from build123d import *

# Parameters (mm, degrees)
SKETCH_R        = 1.4
PAD_DEPTH       = 2
SKETCH001_W     = 86
SKETCH001_H     = 4
PAD001_DEPTH    = 55
FILLET_R        = 2
FILLET001_R     = 2
FILLET002_R     = 1
FILLET003_R     = 1
FILLET004_R     = 1
SKETCH002_R     = 1.4
POCKET_DEPTH    = 5
SKETCH003_W     = 15
SKETCH003_H     = 20
PAD002_DEPTH    = 6.85
SKETCH004_R     = 1.4
POCKET001_DEPTH = 15
SKETCH005_R     = 1.4
POCKET002_DEPTH = 20
SKETCH006_W     = 5
SKETCH006_H     = 5
PAD003_DEPTH    = 5
SKETCH007_R     = 1.4
POCKET003_DEPTH = 5
SKETCH008_R     = 1.4
POCKET004_DEPTH = 5
SKETCH009_R     = 1.4
POCKET005_DEPTH = 4


with BuildPart() as part:
    # Sketch → Pad (new body)
    with BuildSketch(Plane.XY):
        with BuildLine():
            ThreePointArc((-41, 25), (-42.414214, 24.414214), (-43, 23))
            Line((-43, -23), (-43, 23))
            ThreePointArc((-43, -23), (-42.414214, -24.414214), (-41, -25))
            Line((41, -25), (-41, -25))
            ThreePointArc((41, -25), (42.414214, -24.414214), (43, -23))
            Line((43, 23), (43, -23))
            ThreePointArc((43, 23), (42.414214, 24.414214), (41, 25))
            Line((-41, 25), (41, 25))
        make_face()
        with Locations((0, 7)):
            Circle(SKETCH_R, mode=Mode.SUBTRACT)
        with Locations((0, -17)):
            Circle(SKETCH_R, mode=Mode.SUBTRACT)
    extrude(amount=PAD_DEPTH)

    # Sketch001 (on Face12 of Pad) → Pad001 (join)
    with BuildSketch(Plane.XY.offset(2)):
        with Locations((0, 1)):
            Rectangle(SKETCH001_W, SKETCH001_H)
    extrude(amount=PAD001_DEPTH)

    # Fillet
    fillet_edges = [part.edges().sort_by_distance(p)[0] for p in [
        (-43, 1, 57),
    ]]
    fillet(fillet_edges, radius=FILLET_R)

    # Fillet001
    fillet001_edges = [part.edges().sort_by_distance(p)[0] for p in [
        (43, 1, 57),
    ]]
    fillet(fillet001_edges, radius=FILLET001_R)

    # Fillet002
    fillet002_edges = [part.edges().sort_by_distance(p)[0] for p in [
        (-43, 3, 28.5),
    ]]
    fillet(fillet002_edges, radius=FILLET002_R)

    # Fillet003
    fillet003_edges = [part.edges().sort_by_distance(p)[0] for p in [
        (-43, -1, 28.5),
    ]]
    fillet(fillet003_edges, radius=FILLET003_R)

    # Fillet004
    fillet004_edges = [part.edges().sort_by_distance(p)[0] for p in [
        (-43, 0, 0),
    ]]
    fillet(fillet004_edges, radius=FILLET004_R)

    # Sketch002 (on Face12 of Fillet004) → Pocket (cut)
    with BuildSketch(Plane(origin=(0, 3, 0), x_dir=(-1, 0, 0), z_dir=(0, 1, 0))):
        with Locations((-27.5, 24)):
            Circle(SKETCH002_R)
        with Locations((27.5, 24)):
            Circle(SKETCH002_R)
    extrude(amount=-POCKET_DEPTH, mode=Mode.SUBTRACT)

    # Sketch003 (on Face6 of Pocket) → Pad002 (join)
    with BuildSketch(Plane.XY.offset(2)):
        with Locations((-23.5, -11)):
            Rectangle(SKETCH003_W, SKETCH003_H)
        with Locations((23.5, -11)):
            Rectangle(SKETCH003_W, SKETCH003_H)
    extrude(amount=PAD002_DEPTH)

    # Sketch004 (on Face23 of Pad002) → Pocket001 (cut)
    with BuildSketch(Plane(origin=(-31, 0, 0), x_dir=(0, -1, 0), z_dir=(-1, 0, 0))):
        with Locations((6, 5)):
            Circle(SKETCH004_R)
        with Locations((16, 5)):
            Circle(SKETCH004_R)
    extrude(amount=-POCKET001_DEPTH, mode=Mode.SUBTRACT)

    # Sketch005 (on Face28 of Pocket001) → Pocket002 (cut)
    with BuildSketch(Plane.YZ.offset(31)):
        with Locations((-16, 5)):
            Circle(SKETCH005_R)
        with Locations((-6, 5)):
            Circle(SKETCH005_R)
    extrude(amount=-POCKET002_DEPTH, mode=Mode.SUBTRACT)

    # Sketch006 (on Face6 of Pocket002) → Pad003 (join)
    with BuildSketch(Plane.XY.offset(2)):
        with Locations((-7.5, -18.5)):
            Rectangle(SKETCH006_W, SKETCH006_H)
        with Locations((7.5, -18.5)):
            Rectangle(SKETCH006_W, SKETCH006_H)
    extrude(amount=PAD003_DEPTH)

    # Sketch007 (on Face30 of Pad003) → Pocket003 (cut)
    with BuildSketch(Plane.XZ.offset(21)):
        with Locations((-7.5, 4.5)):
            Circle(SKETCH007_R)
    extrude(amount=-POCKET003_DEPTH, mode=Mode.SUBTRACT)

    # Sketch008 (on Face34 of Pocket003) → Pocket004 (cut)
    with BuildSketch(Plane.XZ.offset(21)):
        with Locations((7.5, 4.5)):
            Circle(SKETCH008_R)
    extrude(amount=-POCKET004_DEPTH, mode=Mode.SUBTRACT)

    # Sketch009 (on Face20 of Pocket004) → Pocket005 (cut)
    with BuildSketch(Plane.XZ.offset(1)):
        with Locations((-7.5, 52.5)):
            Circle(SKETCH009_R)
        with Locations((7.5, 52.5)):
            Circle(SKETCH009_R)
    extrude(amount=-POCKET005_DEPTH, mode=Mode.SUBTRACT)


solid = part.part
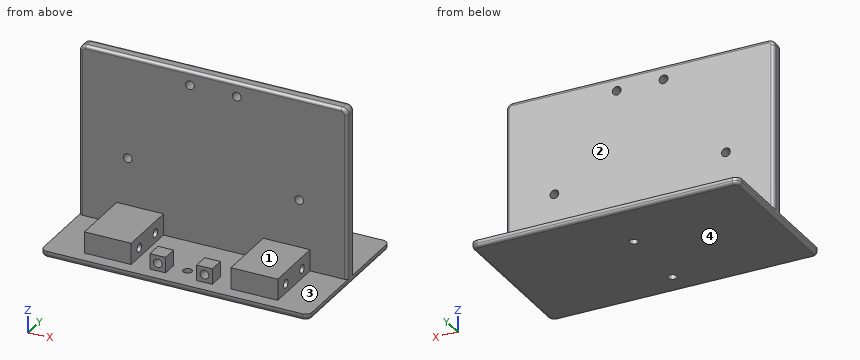
Design review of the part built by this model. Coordinates are the model's own, in mm. Face numbers are marked on the shaded views. A direction names the side the tool comes from. Round coordinates to 2 decimals unless told otherwise and drop trailing zeros. Write each loop counter-clockwise with the first axis right and the second up, starting at its lowest first coordinate (ties: lowest second). Pieces come first, ordered by that corner, then holes.
Item 1: Consider section A-A on x = 27.5. Give the boundary of the cut face in (y, z), and give its area (3 significant figures).
Item 2: For pin 1 Ø3.5 at (x, z) = (-21, 7) entering from -Y; pin 2 Ø3 at (x, z) = (2, 10) entering from +Y; pin 3 Ø5.5 at (x, y) = (-7.5, -18.5) entering from +Z, all flat-tipped, find the tip position at first contact; note any pin that passes through.
Item 3: Consider section D-D on x = -18. Give the boundary of the cut face in (y, z), and give its area (3 significant figures).
Item 4: Draft analysis for pull direction X (two halves, no side actions). For the marked faces 3 and 4, state which applies: released by +X, released by -X, zero draft, split by the parting line, or undercut.
Item 5: Consider section B-B on z = 24. Give the boundary of the cut face in (x, y).
Item 6: Wall thickness on L1, parallel to X at y = -14, z = 7; L2, parallel to X at y = -19, z = 4; L3, parallel to Z at x = 35, y = -8.5: over which ranges is each line inside the solid? List them lowest first.
Item 7: Consider section C-C on y = 7. Give the boundary of the cut face in (x, z).
Item 8: For the marked faces 1 and 2, list the 3-axis set-ups (+Z, -Z, +X, -X, +Y, -Y) from which the entire face can be reached by the end or side of a thin tool; tool diameter is ignored.
Check values:
1. outline: (-25, 1) arc R1 ccw to (-24, 0) - (24, 0) arc R1 ccw to (25, 1) - (25, 2) - (3, 2) - (3, 22.6) - (-1, 22.6) - (-1, 8.85) - (-21, 8.85) - (-21, 2) - (-25, 2) - close; (-1, 25.4) - (3, 25.4) - (3, 56) arc R1 ccw to (2, 57) - (0, 57) arc R1 ccw to (-1, 56) - close; hole circle Ø2.8 at (-16, 5); hole circle Ø2.8 at (-6, 5)
1. area: 433 mm2
2. pin 1: stops at y = -21
2. pin 2: stops at y = 3
2. pin 3: stops at z = 7
3. outline: (-25, 1) arc R1 ccw to (-24, 0) - (24, 0) arc R1 ccw to (25, 1) - (25, 2) - (3, 2) - (3, 56) arc R1 ccw to (2, 57) - (0, 57) arc R1 ccw to (-1, 56) - (-1, 8.85) - (-21, 8.85) - (-21, 2) - (-25, 2) - close; hole circle Ø2.8 at (-16, 5); hole circle Ø2.8 at (-6, 5)
3. area: 444 mm2
4. face 3: undercut
4. face 4: zero draft
5. outline: (-43, 0) arc R1 ccw to (-42, -1) - (-28.9, -1) - (-28.9, 3) - (-42, 3) arc R1 ccw to (-43, 2) - close; (-26.1, -1) - (26.1, -1) - (26.1, 3) - (-26.1, 3) - close; (28.9, -1) - (42, -1) arc R1 ccw to (43, 0) - (43, 2) arc R1 ccw to (42, 3) - (28.9, 3) - close
6. L1: x = -31 to -16, 16 to 31
6. L2: x = -31 to -16, -10 to -8.81, -6.19 to -5, 5 to 6.19, 8.81 to 10, 16 to 31
6. L3: z = 0 to 2
7. outline: (-43, 1) arc R1 ccw to (-42, 0) - (-1.4, 0) - (-1.4, 2) - (-43, 2) - close; (1.4, 0) - (42, 0) arc R1 ccw to (43, 1) - (43, 2) - (1.4, 2) - close
8. face 1: +Z, +X, -X, -Y
8. face 2: +Z, +X, -X, +Y
